Autodesk Inventor part; units mm, degrees
ref_plane "YZ Plane" through (0, 0, 0) normal (1, 0, 0) x (0, 1, 0)
ref_plane "XZ Plane" through (0, 0, 0) normal (0, 1, 0) x (-1, 0, 0)
ref_plane "XY Plane" through (0, 0, 0) normal (0, 0, 1) x (1, 0, 0)
sketch "Sketch1" plane through (0, 0, 0) normal (0, 0, 1) x (1, 0, 0)
  line L0 (-10, 25) -> (10, 25)
  line L1 (13, 28) -> (-13, 28)
  line L2 (-13, 28) -> (-13, 3)
  line L3 (13, 3) -> (13, 28)
  line L4 (11, 0) -> (17, 0)
  line L5 (17, 3) -> (13, 3)
  line L6 (-13, 3) -> (-17, 3)
  line L7 (-17, 0) -> (-11, 0)
  line L8 (-17, 3) -> (-19, 3)
  line L9 (-19, 3) -> (-19, 0)
  line L10 (-19, 0) -> (-17, 0)
  line L11 (17, 0) -> (19, 0)
  line L12 (19, 0) -> (19, 3)
  line L13 (17, 3) -> (19, 3)
  line L14 (-10, 25) -> (-11, 25)
  line L15 (-11, 25) -> (-11, 0)
  line L16 (10, 25) -> (11, 25)
  line L17 (11, 25) -> (11, 0)
  point P0 (0, 0)
  dimension "d0" = 20
  dimension "d2" = 3
  dimension "d12" = 3
  dimension "d17" = 1
extrude "Extrusion1" add sketch "Sketch1" along normal blind 5
sketch "Sketch2" plane through (-19, 3, 0) normal (0, 1, 0) x (1, 0, 0)
  circle A0 centre (3, -2.5) radius 1.5
  point P0 (19, 0)
  dimension "d13" = 3
extrude "Extrusion2" cut sketch "Sketch2" against normal up to next
sketch "Sketch3" plane through (-13, 28, 0) normal (0, 1, 0) x (1, 0, 0)
  point P0 (13, 0)
mirror "Mirror1" about plane through (0, 0, 0) normal (1, 0, 0) of "Extrusion2"
sketch "Sketch4" plane through (-19, 0, 0) normal (0, -1, 0) x (1, 0, 0)
  point P0 (19, 0)
properties part number "servo shaft"
The listing builds one solid part. Answer for the finished solid, in the listing's coordinates (mm). A direction names the side the tool comes from. Round coordinates to 2 decimals unless told otherwise and drop trailing zeros. Write each loop counter-clockwise with the first axis right and the second up, starting at its lowest first coordinate (ties: lowest second). Pieces come first, ordered by that corner, then holes. Notation, with made-up numbers: (71.25, 33.25) -> (75.25, 33.25) arc R13 ccw to (75.25, 49.25) -> close; hole circle Ø1 at (38, 12.5). An arc over 180 degrees is marked (long way). Use CSV: the item, a comma, the result in double quotes. Start each with the question number.
(1) Consider L1, parallel to X at y = 1.35, z = 2.5; L2, parallel to X at y = 4.75, z = 1.8; L3, parallel to Z at x = -16, y = 2. Determine where each line is inside the solid, lowest interval first. Write a range as from..to.
(2) Section A-A on y = 7.75 is taken. Give the vertices of the cut face in (x, z).
(3) Section D-D on x = -9 is taken. Give the vertices of the cut face in (y, z).
(4) Each of these flat-tipped pins is pushed along its axis until it touches: pin 1 (1 mm diameter, centred on x = -3.5, z = 1, fed in from -Y); pin 2 (12 mm diameter, centred on x = 7, y = 5, fed in from +Z); pin 3 (1.5 mm diameter, centred on y = 18.5, z = 2.5, fed in from +X); pin 4 (1.5 mm diameter, centred on y = 21, z = 2.5, fed in from -X). Where does it stop, or does it pass through?
(5) Section C-C on z = 2.5 is taken. Give the vertices of the cut face in (x, y), then the cut area to 3 significant figures.
(6) The mould has two halves that part along Z. Classify faces 6 (the face through (-0.1, 25.5, 0)), 7 (the face through (11, 13, 2)), 8 (the face through (-17.5, 1.52, 2.43)): released by +Z, released by -Z, zero draft, split by the parting line, or undercut.
(7) Section B-B on x = 16 is taken. Give the vertices of the cut face in (y, z), then the cut area to 3 significant figures.
(8) Which of the six approach directions +Z, -Z, +X, -X, +Y, -Y give full straight-line access (tool end or side, diameter ignored) to faces 1 (the face through (-13, 16, 2)), 2 (the face through (13, 15, 2)), 3 (the face through (0, 28, 2)), 4 (the face through (-0.1, 25.5, 5)), 5 (the face through (0, 25, 2))?
A:
1,L1,"x = -19..-17.5, -14.5..-11, 11..14.5, 17.5..19"
1,L2,"x = -13..-11, 11..13"
1,L3,"z = 0..1, 4..5"
2,outline,"(-13, 0) -> (-11, 0) -> (-11, 5) -> (-13, 5) -> close; (11, 0) -> (13, 0) -> (13, 5) -> (11, 5) -> close"
3,outline,"(25, 0) -> (28, 0) -> (28, 5) -> (25, 5) -> close"
4,pin 1,"stops at y = 25"
4,pin 2,"stops at z = 5"
4,pin 3,"stops at x = 13"
4,pin 4,"stops at x = -13"
5,outline,"(-19, 0) -> (-17.5, 0) -> (-17.5, 3) -> (-19, 3) -> close; (-14.5, 0) -> (-11, 0) -> (-11, 25) -> (11, 25) -> (11, 0) -> (14.5, 0) -> (14.5, 3) -> (13, 3) -> (13, 28) -> (-13, 28) -> (-13, 3) -> (-14.5, 3) -> close; (17.5, 0) -> (19, 0) -> (19, 3) -> (17.5, 3) -> close"
5,area,"196 mm²"
6,face 6,"released by -Z"
6,face 7,"zero draft"
6,face 8,"undercut"
7,outline,"(0, 0) -> (3, 0) -> (3, 1) -> (0, 1) -> close; (0, 4) -> (3, 4) -> (3, 5) -> (0, 5) -> close"
7,area,"6.00 mm²"
8,face 1,"+Z, -Z, -X, +Y"
8,face 2,"+Z, -Z, +X, +Y"
8,face 3,"+Z, -Z, +X, -X, +Y"
8,face 4,"+Z, +X, -X, +Y, -Y"
8,face 5,"+Z, -Z, -Y"
